Source: CAD feature listing. Evaluate the final solid. Frame: model axes, mm. A direction names the side the tool comes from. Round coordinates to 2 decimals unless told otherwise and drop trailing zeros. Write each loop counter-clockwise with the first axis right and the second up, starting at its lowest first coordinate (ties: lowest second). Pieces come first, ordered by that corner, then holes. Notation, with made-up numbers: M -16.75,87.25 L 12.25,87.25 A14 cw 12.25,108.25 Z; hole C -30,32 d4. An arc over 180 degrees is marked long. Answer in a Markdown table with one row per item.
from build123d import *

# Parameters (mm, degrees)
F3_DEPTH  = 90
F4_DEPTH  = 40
F5_DEPTH  = 30
F6_W      = 20
F6_H      = 12
F7_DEPTH  = 120.001
F9_DEPTH  = 33
F8_R      = 8
F10_DEPTH = 120.001
F12_DEPTH = 30


with BuildPart() as f3:
    # F2 (on Right) → F3 (new body)
    with BuildSketch(Plane.YZ):
        Polygon((-60, -22), (-60, -42), (60, -42), (60, -22), (-15.6524758425, -22), align=None)
        with BuildLine():
            Line((-60, 78), (-60, -22))
            Line((-60, -22), (-15.6524758425, -22))
            ThreePointArc((-15.6524758425, -22), (-23.9960084988, -12.3770584602), (-27, 0))
            Line((-27, 0), (-27, 78))
            Line((-27, 78), (-60, 78))
        make_face()
        with BuildLine():
            Line((-15.6524758425, -22), (60, -22))
            Line((60, -22), (60, 10))
            ThreePointArc((60, 10), (48.5108747069, 12.0645834035), (38.4593407715, 18))
            Line((38.4593407715, 18), (27, 18))
            Line((27, 18), (27, 78))
            Line((27, 78), (20, 78))
            ThreePointArc((20, 78), (15.4919333848, 65.3508893593), (4, 58.4040820577))
            Line((4, 58.4040820577), (4, 15.4919333848))
            ThreePointArc((4, 15.4919333848), (0, -16), (-4, 15.4919333848))
            Line((-4, 15.4919333848), (-4, 58.4040820577))
            ThreePointArc((-4, 58.4040820577), (-15.4919333848, 65.3508893593), (-20, 78))
            Line((-20, 78), (-27, 78))
            Line((-27, 78), (-27, 0))
            ThreePointArc((-27, 0), (-23.9960084988, -12.3770584602), (-15.6524758425, -22))
        make_face()
    extrude(amount=-F3_DEPTH)

    # F2 (on Right) → F4 (cut)
    with BuildSketch(Plane.YZ):
        Polygon((-60, -22), (-60, -42), (60, -42), (60, -22), (-15.6524758425, -22), align=None)
    extrude(amount=-F4_DEPTH, mode=Mode.SUBTRACT)

    # F2 (on Right) → F5 (cut)
    with BuildSketch(Plane.YZ):
        with BuildLine():
            Line((-60, 78), (-60, -22))
            Line((-60, -22), (-15.6524758425, -22))
            ThreePointArc((-15.6524758425, -22), (-23.9960084988, -12.3770584602), (-27, 0))
            Line((-27, 0), (-27, 78))
            Line((-27, 78), (-60, 78))
        make_face()
    extrude(amount=-F5_DEPTH, mode=Mode.SUBTRACT)

    # F6 (on face) → F7 (cut, through all)
    with BuildSketch(Plane(origin=(0, 60, 0), x_dir=(-1, 0, 0), z_dir=(0, 1, 0))):
        with Locations((70, -36)):
            Rectangle(F6_W, F6_H)
    extrude(amount=-F7_DEPTH, mode=Mode.SUBTRACT)

    # F8 (on face) → F9 (cut)
    with BuildSketch(Plane.XZ.offset(60)):
        with BuildLine():
            ThreePointArc((-60, 43), (-45, 58), (-30, 43))
            Line((-30, 43), (-30, 78))
            Line((-30, 78), (-90, 78))
            Line((-90, 78), (-90, 10))
            Line((-90, 10), (-60, 10))
            Line((-60, 10), (-60, 43))
        make_face()
    extrude(amount=-F9_DEPTH, mode=Mode.SUBTRACT)

    # F8 (on face) → F10 (cut, through all)
    with BuildSketch(Plane.XZ.offset(60)):
        with Locations((-45, 43)):
            Circle(F8_R)
    extrude(amount=-F10_DEPTH, mode=Mode.SUBTRACT)

    # F11 (on face) → F12 (join, through all)
    with BuildSketch(Plane(origin=(-90, 0, 0), x_dir=(0, -1, 0), z_dir=(-1, 0, 0))):
        with BuildLine():
            ThreePointArc((60, 10), (36.6654762208, 19.6654762208), (27, 43))
            Line((27, 43), (27, 10))
            Line((27, 10), (60, 10))
        make_face()
    extrude(amount=-F12_DEPTH)


solid = f3.part
Q1. Access query for faces 4 (the flat face through (-34, -27, 56)), 5 (the flat face through (-70, 1, -30)), 6 (the cylindrical face through (-14.79, -23.91, -12.54)), 7 (the cylindrical face through (-44.37, 15.61, 65.5)). Directions: +Z, -Z, +X, -X, +Y, -Y. A direction counts if a zero-diameter tool reaches every point of the face in a straight line with its end or side. Return the directions, or none.
Solutions:
| item | result |
|---|---|
| face 4 | +Z, -Y |
| face 5 | -Z, +Y, -Y |
| face 6 | -Z, +X, -Y |
| face 7 | +Z, +X, -X |
Q2. Section C-C (x = -45). Return loops of the section in (y, z), and give its area (3 significant figures).
Solutions:
| item | result |
|---|---|
| outline | M -60,-42 L 60,-42 L 60,10 A33 cw 38.46,18 L 27,18 L 27,35 L 4,35 L 4,15.49 A16 cw long -4,15.49 L -4,35 L -60,35 Z; M -60,51 L -4,51 L -4,58.4 A20 cw -20,78 L -27,78 L -27,58 L -60,58 Z; M 4,51 L 27,51 L 27,78 L 20,78 A20 cw 4,58.4 Z |
| area | 8,610 mm2 |
Q3. Section A-A (y = 0). Return loops of the section in (x, z).
Solutions:
| item | result |
|---|---|
| outline | M -90,-42 L -80,-42 L -80,-30 L -60,-30 L -60,-42 L -40,-42 L -40,-22 L 0,-22 L 0,-16 L -90,-16 Z |
Q4. Section D-D (z = 37). Return loops of the section in (x, y), and give its area (3 significant figures).
Solutions:
| item | result |
|---|---|
| outline | M -90,-27.55 L -60,-27.55 L -60,-60 L -50.29,-60 L -50.29,-4 L -90,-4 Z; M -90,4 L -50.29,4 L -50.29,27 L -90,27 Z; M -39.71,-60 L -30,-60 L -30,-27 L 0,-27 L 0,-4 L -39.71,-4 Z; M -39.71,4 L 0,4 L 0,27 L -39.71,27 Z |
| area | 4,310 mm2 |
Q5. Pull-direction query (Z, two-part tool) for faces 1 (the flat face through (-44, -23, 78)), 2 (the cylindrical face through (-50.9, 15.3, 48.4)), 3 (the flat face through (-60, -60, -2)); classes: pulls with the +Z half, pulls with the -Z half, needs draft (parallel to the pull), parting line crosses it, or undercut.
Solutions:
| item | result |
|---|---|
| face 1 | pulls with the +Z half |
| face 2 | undercut |
| face 3 | needs draft |
Q6. Contact query for flat-ended pins moving along their axis: pin 1 Ø6 at (x, y) = (-73.5, -14.5) entering from -Z; pin 2 Ø8 at (x, z) = (-17.5, -8.5) entering from -Y; pin 3 Ø9.5 at (x, z) = (-45, 43) entering from +Y; pin 4 Ø10 at (y, z) = (-48, 34.5) entering from -X. Output: stop coordinate, or through.
Solutions:
| item | result |
|---|---|
| pin 1 | stops at z = -30 |
| pin 2 | stops at y = -26.62 |
| pin 3 | passes through |
| pin 4 | stops at x = -60 |
Q7. Section B-B (z = 54.5). Return loops of the section in (x, y).
Solutions:
| item | result |
|---|---|
| outline | M -90,-27 L -54.63,-27 L -54.63,-60 L -35.37,-60 L -35.37,-27 L 0,-27 L 0,-4 L -90,-4 Z; M -90,4 L 0,4 L 0,27 L -90,27 Z |
Q8. Material intervals for probe 1 along Y at (x, z) = (-40, 51); probe 2 along Y at (x, z) = (-29.5, 25.5); probe 3 along Z at (x, y) = (-45, 10.5), sorted ascending.
Solutions:
| item | result |
|---|---|
| probe 1 | y = -60 to -4, 4 to 27 |
| probe 2 | y = -27 to -4, 4 to 27 |
| probe 3 | z = -42 to -12.07, 12.07 to 35, 51 to 60.98 |
